```python
from build123d import *

# Parameters (mm, degrees)
BOSS_EXTRUDE3_DEPTH      = 6.35
FILLET1_R                = 6.35
CIRPATTERN5_COUNT        = 4
FILLET1_OF_CIRPATTERN5_R = 6.35
BOSS_EXTRUDE4_DEPTH      = 6.35
CIRPATTERN4_COUNT        = 4
SKETCH6_R                = 234.193665804
SKETCH6_R_2              = 215.9
CUT_EXTRUDE1_DEPTH       = 350.00288517
FILLET2_R                = 0.635
SKETCH7_R                = 60.93897947
CUT_EXTRUDE2_DEPTH       = 4.953
SKETCH8_R                = 79.670197019
CUT_EXTRUDE3_DEPTH       = 18.9484
CUT_EXTRUDE4_START       = 20.32
SKETCH11_R               = 219.71
SKETCH11_R_2             = 50.8
CUT_EXTRUDE4_DEPTH       = 20.32
CUT_EXTRUDE10_REACH      = 337.887
SKETCH20_R               = 30.226
SKETCH20_R_2             = 26.8224
CUT_EXTRUDE11_DEPTH      = 2.0066
CUT_EXTRUDE13_DEPTH      = 3.175
CIRPATTERN6_COUNT        = 8
SKETCH24_W               = 27.0002
SKETCH24_H               = 10.092146942
SKETCH25_R               = 27.9527
CUT_EXTRUDE14_DEPTH      = 14.3002


with BuildPart() as part:
    # Sketch1 → Revolve2 (revolve)
    with BuildSketch(Plane.XY, mode=Mode.PRIVATE) as revolve2_sk:
        with BuildLine():
            Line((-140.081298787, 50.8), (-140.081298787, 0))
            Line((-140.081298787, 0), (-39.979898787, 0))
            Line((-39.979898787, 0), (-39.979898787, 46.736))
            Line((-39.979898787, 46.736), (-43.154898787, 46.736))
            ThreePointArc((-43.154898787, 46.736), (-47.645026847, 48.595871939), (-49.504898787, 53.086))
            Line((-49.504898787, 53.086), (-49.504898787, 219.71))
            Line((-49.504898787, 219.71), (-64.998898787, 219.71))
            Line((-64.998898787, 219.71), (-64.998898787, 63.5))
            ThreePointArc((-64.998898787, 63.5), (-68.718642666, 54.519743879), (-77.698898787, 50.8))
            Line((-77.698898787, 50.8), (-140.081298787, 50.8))
        make_face()
        with BuildLine():
            Line((-9.677698787, 219.71), (-17.678698787, 219.71))
            Line((-17.678698787, 219.71), (-17.678698787, 77.7875))
            Line((-17.678698787, 77.7875), (1.650701213, 77.7875))
            Line((1.650701213, 77.7875), (18.846501213, 77.7875))
            Line((18.846501213, 77.7875), (18.846501213, 93.599))
            ThreePointArc((18.846501213, 93.599), (18.400131948, 94.676630735), (17.322501213, 95.123))
            Line((17.322501213, 95.123), (-6.629698787, 95.123))
            ThreePointArc((-6.629698787, 95.123), (-7.707329521, 95.569369265), (-8.153698787, 96.647))
            Line((-8.153698787, 96.647), (-8.153698787, 218.186))
            ThreePointArc((-8.153698787, 218.186), (-8.600068052, 219.263630735), (-9.677698787, 219.71))
        make_face()
    revolve(revolve2_sk.sketch.rotate(Axis((-140.081298787, 0, 0), (1, 0, 0)), 180), axis=Axis((-140.081298787, 0, 0), (1, 0, 0)))

    # Sketch4 → Boss-Extrude3 (add, symmetric)
    with BuildSketch(Plane(origin=(0, 0, 0), x_dir=(1, 0, 0), z_dir=(0, -0.7071067811865488, 0.7071067811865464))):
        Polygon((-17.678698787, 219.71), (-30.378698787, 219.71), (-30.378698787, 130.302), (-36.804898787, 130.302), (-36.804898787, 219.71), (-49.504898787, 219.71), (-49.504898787, 77.7875), (-17.678698787, 77.7875), align=None)
    boss_extrude3 = extrude(amount=BOSS_EXTRUDE3_DEPTH, both=True)

    # Fillet1
    # the kernel refuses this fillet: 6.35 mm, written as the material it takes off along each edge
    with BuildSketch(Plane(origin=(-30.378698787, 87.647299742, 96.627555863), x_dir=(0, -0.7071067811865464, -0.7071067811865486), z_dir=(-1, 0, 0))) as fillet1_piece_1:
        with BuildLine():
            CenterArc((FILLET1_R, -FILLET1_R), FILLET1_R, 90, 90)
            Line((0, -FILLET1_R), (0, 0))
            Line((0, 0), (FILLET1_R, 0))
        make_face()
    extrude(amount=6.4262, mode=Mode.SUBTRACT)
    with BuildSketch(Plane(origin=(-30.378698787, 96.627555863, 87.647299742), x_dir=(0, -0.7071067811865464, -0.7071067811865486), z_dir=(-1, 0, 0))) as fillet1_piece_2:
        with BuildLine():
            CenterArc((FILLET1_R, FILLET1_R), FILLET1_R, 180, 90)
            Line((0, FILLET1_R), (0, 0))
            Line((0, 0), (FILLET1_R, 0))
        make_face()
    extrude(amount=6.4262, mode=Mode.SUBTRACT)
    with BuildSketch(Plane(origin=(-49.504898787, 59.494196802, 50.513940681), x_dir=(0, 0.707106781186547, 0.7071067811865481), z_dir=(1, 0, 0)), Plane(origin=(-49.504898787, 50.513940681, 59.494196802), x_dir=(0, 0.7071067811865492, -0.7071067811865459), z_dir=(1, 0, 0))) as fillet1_piece_3:
        with BuildLine():
            CenterArc((FILLET1_R, FILLET1_R), FILLET1_R, 180, 90)
            Line((0, FILLET1_R), (0, 0))
            Line((0, 0), (FILLET1_R, 0))
        make_face()
    extrude(amount=31.8262, mode=Mode.SUBTRACT)

    # CirPattern5: Boss-Extrude3 ×4 about axis
    cirpattern5_axis = Axis((0, 0, 0), (1, 0, 0))
    for i in range(1, CIRPATTERN5_COUNT):
        add(boss_extrude3.rotate(cirpattern5_axis, i * 360 / CIRPATTERN5_COUNT))

    # Fillet1 of CirPattern5
    # the kernel refuses this fillet: 6.35 mm, written as the material it takes off along each edge
    with BuildSketch(Plane(origin=(-30.378698787, -96.627555863, 87.647299742), x_dir=(0, 0.7071067811865509, -0.7071067811865441), z_dir=(-1, 0, 0)), Plane(origin=(-30.378698787, -87.647299742, -96.627555863), x_dir=(0, 0.7071067811865452, 0.7071067811865498), z_dir=(-1, 0, 0)), Plane(origin=(-30.378698787, 96.627555863, -87.647299742), x_dir=(0, -0.7071067811865498, 0.7071067811865454), z_dir=(-1, 0, 0))) as fillet1_of_cirpattern5_piece_1:
        with BuildLine():
            CenterArc((FILLET1_OF_CIRPATTERN5_R, -FILLET1_OF_CIRPATTERN5_R), FILLET1_OF_CIRPATTERN5_R, 90, 90)
            Line((0, -FILLET1_OF_CIRPATTERN5_R), (0, 0))
            Line((0, 0), (FILLET1_OF_CIRPATTERN5_R, 0))
        make_face()
    extrude(amount=6.4262, mode=Mode.SUBTRACT)
    with BuildSketch(Plane(origin=(-30.378698787, -87.647299742, 96.627555863), x_dir=(0, 0.7071067811865509, -0.7071067811865441), z_dir=(-1, 0, 0)), Plane(origin=(-30.378698787, -96.627555863, -87.647299742), x_dir=(0, 0.7071067811865441, 0.7071067811865509), z_dir=(-1, 0, 0)), Plane(origin=(-30.378698787, 87.647299742, -96.627555863), x_dir=(0, -0.7071067811865509, 0.7071067811865441), z_dir=(-1, 0, 0))) as fillet1_of_cirpattern5_piece_2:
        with BuildLine():
            CenterArc((FILLET1_OF_CIRPATTERN5_R, FILLET1_OF_CIRPATTERN5_R), FILLET1_OF_CIRPATTERN5_R, 180, 90)
            Line((0, FILLET1_OF_CIRPATTERN5_R), (0, 0))
            Line((0, 0), (FILLET1_OF_CIRPATTERN5_R, 0))
        make_face()
    extrude(amount=6.4262, mode=Mode.SUBTRACT)
    with BuildSketch(Plane(origin=(-49.504898787, -50.513940681, 59.494196802), x_dir=(0, -0.7071067811865475, 0.7071067811865475), z_dir=(1, 0, 0)), Plane(origin=(-49.504898787, -59.494196802, 50.513940681), x_dir=(0, 0.7071067811865464, 0.7071067811865486), z_dir=(1, 0, 0)), Plane(origin=(-49.504898787, -59.494196802, -50.513940681), x_dir=(0, -0.7071067811865481, -0.707106781186547), z_dir=(1, 0, 0)), Plane(origin=(-49.504898787, -50.513940681, -59.494196802), x_dir=(0, -0.7071067811865486, 0.7071067811865464), z_dir=(1, 0, 0)), Plane(origin=(-49.504898787, 50.513940681, -59.494196802), x_dir=(0, 0.7071067811865476, -0.7071067811865476), z_dir=(1, 0, 0)), Plane(origin=(-49.504898787, 59.494196802, -50.513940681), x_dir=(0, -0.7071067811865459, -0.7071067811865492), z_dir=(1, 0, 0))) as fillet1_of_cirpattern5_piece_3:
        with BuildLine():
            CenterArc((FILLET1_OF_CIRPATTERN5_R, FILLET1_OF_CIRPATTERN5_R), FILLET1_OF_CIRPATTERN5_R, 180, 90)
            Line((0, FILLET1_OF_CIRPATTERN5_R), (0, 0))
            Line((0, 0), (FILLET1_OF_CIRPATTERN5_R, 0))
        make_face()
    extrude(amount=31.8262, mode=Mode.SUBTRACT)

    # Sketch5 → Boss-Extrude4 (add, symmetric)
    with BuildSketch(Plane(origin=(0, 0, 0), x_dir=(-1, 0, 0), z_dir=(0, 0, -1))):
        Polygon((49.504898787, 219.71), (49.504898787, 73.66), (36.804898787, 86.36), (36.804898787, 219.71), align=None)
        Polygon((17.678698787, 77.7875), (17.678698787, 219.71), (30.378698787, 219.71), (30.378698787, 90.4875), align=None)
    boss_extrude4 = extrude(amount=BOSS_EXTRUDE4_DEPTH, both=True)

    # CirPattern4: Boss-Extrude4 ×4 about axis
    cirpattern4_axis = Axis((0, 0, 0), (1, 0, 0))
    for i in range(1, CIRPATTERN4_COUNT):
        add(boss_extrude4.rotate(cirpattern4_axis, i * 360 / CIRPATTERN4_COUNT))

    # Sketch6 → Cut-Extrude1 (cut, through all)
    with BuildSketch(Plane.ZY.offset(140.081298787)):
        Circle(SKETCH6_R)
        with Locations(Location((0, 0, 0), (0, 0, 270))):
            Circle(SKETCH6_R_2, mode=Mode.SUBTRACT)
    extrude(amount=-CUT_EXTRUDE1_DEPTH, mode=Mode.SUBTRACT)

    # Fillet2
    fillet2_edges = [part.edges().sort_by_distance(p)[0] for p in [
        (-39.979898787, 46.736, 0),
    ]]
    fillet(fillet2_edges, radius=FILLET2_R)

    # Sketch7 → Cut-Extrude2 (cut)
    with BuildSketch(Plane(origin=(-39.979898787, 0, 0), x_dir=(0, 0, -1), z_dir=(1, 0, 0))):
        Circle(SKETCH7_R)
    extrude(amount=-CUT_EXTRUDE2_DEPTH, mode=Mode.SUBTRACT)

    # Sketch8 → Cut-Extrude3 (cut)
    with BuildSketch(Plane.ZY.offset(140.081298787)):
        Circle(SKETCH8_R)
    extrude(amount=-CUT_EXTRUDE3_DEPTH, mode=Mode.SUBTRACT)

    # Sketch11 → Cut-Extrude4 (cut)
    with BuildSketch(Plane.ZY.offset(64.998898787).offset(CUT_EXTRUDE4_START)):
        Circle(SKETCH11_R)
        with Locations(Location((0, 0, 0), (0, 0, 270))):
            Circle(SKETCH11_R_2, mode=Mode.SUBTRACT)
    extrude(amount=-CUT_EXTRUDE4_DEPTH, mode=Mode.SUBTRACT)

    # Sketch12 → Cut-Revolve1 (revolve, cut)
    with BuildSketch(Plane(origin=(0, 0, 0), x_dir=(1, 0, 0), z_dir=(0, 1, 0)), mode=Mode.PRIVATE) as cut_revolve1_sk:
        with BuildLine():
            Line((-121.132898787, 31.75), (-80.111898787, 31.75))
            ThreePointArc((-80.111898787, 31.75), (-76.957987839, 32.588616713), (-74.637123327, 34.882961973))
            Line((-74.637123327, 34.882961973), (-65.874123327, 49.795890249))
            ThreePointArc((-65.874123327, 49.795890249), (-65.613530636, 50.287482958), (-65.396970658, 50.8))
            Line((-65.396970658, 50.8), (-121.132898787, 50.8))
            Line((-121.132898787, 50.8), (-121.132898787, 31.75))
        make_face()
    revolve(cut_revolve1_sk.sketch.rotate(Axis((-60.172898787, 0, 0), (-1, 0, 0)), 270), axis=Axis((-60.172898787, 0, 0), (-1, 0, 0)), mode=Mode.SUBTRACT)

    # Sketch18 → Cut-Extrude10 (cut, up to next)
    with BuildSketch(Plane.ZY.offset(121.132898787), mode=Mode.PRIVATE) as cut_extrude10_sk1:
        with BuildLine():
            Line((-14.359429538, -21.094621628), (-21.094621628, -14.359429538))
            Line((-21.094621628, -14.359429538), (-17.575856913, -10.840664823))
            ThreePointArc((-17.575856913, -10.840664823), (14.601896453, 14.601896453), (-10.840664823, -17.575856913))
            Line((-10.840664823, -17.575856913), (-14.359429538, -21.094621628))
        make_face()
    cut_extrude10_tool1 = extrude(cut_extrude10_sk1.sketch, amount=-CUT_EXTRUDE10_REACH, mode=Mode.PRIVATE) & part.part
    add(cut_extrude10_tool1.solids().sort_by_distance((-121.132899, -0.51024, -0.51024))[0], mode=Mode.SUBTRACT)

    # Sketch20 → Cut-Extrude11 (cut)
    with BuildSketch(Plane.ZY.offset(121.132898787)):
        with Locations(Location((0, 0, 0), (0, 0, 270))):
            Circle(SKETCH20_R)
        with Locations(Location((0, 0, 0), (0, 0, 270))):
            Circle(SKETCH20_R_2, mode=Mode.SUBTRACT)
    extrude(amount=-CUT_EXTRUDE11_DEPTH, mode=Mode.SUBTRACT)

    # Sketch22 → Cut-Extrude13 (cut)
    with BuildSketch(Plane.ZY.offset(64.998898787)):
        with BuildLine():
            Line((50.92871008, 64.399094261), (145.78051919, 159.250903372))
            ThreePointArc((145.78051919, 159.250903372), (82.621353048, 199.465591069), (9.525, 215.689787368))
            Line((9.525, 215.689787368), (9.525, 84.123223233))
            ThreePointArc((9.525, 84.123223233), (24.00104092, 61.192302667), (50.92871008, 64.399094261))
        make_face()
    cut_extrude13 = extrude(amount=-CUT_EXTRUDE13_DEPTH, mode=Mode.SUBTRACT)

    # CirPattern6: Cut-Extrude13 ×8 about axis
    cirpattern6_axis = Axis((0, 0, 0), (1, 0, 0))
    for i in range(1, CIRPATTERN6_COUNT):
        add(cut_extrude13.rotate(cirpattern6_axis, i * 360 / CIRPATTERN6_COUNT), mode=Mode.SUBTRACT)

    # Sketch24 → Cut-Revolve2 (revolve, cut)
    with BuildSketch(Plane(origin=(0, 0, 0), x_dir=(1, 0, 0), z_dir=(0, 1, 0)), mode=Mode.PRIVATE) as cut_revolve2_sk:
        with Locations((5.346401213, 95.533573471)):
            Rectangle(SKETCH24_W, SKETCH24_H)
    revolve(cut_revolve2_sk.sketch.rotate(Axis((-154.951085714, 0, 0), (1, 0, 0)), 271.68541304), axis=Axis((-154.951085714, 0, 0), (1, 0, 0)), mode=Mode.SUBTRACT)

    # Sketch25 → Cut-Extrude14 (cut)
    with BuildSketch(Plane(origin=(-44.932898787, 0, 0), x_dir=(0, 0, -1), z_dir=(1, 0, 0))):
        with Locations(Location((0, 0, 0), (0, 0, 90))):
            Circle(SKETCH25_R)
    extrude(amount=-CUT_EXTRUDE14_DEPTH, mode=Mode.SUBTRACT)


solid = part.part
```
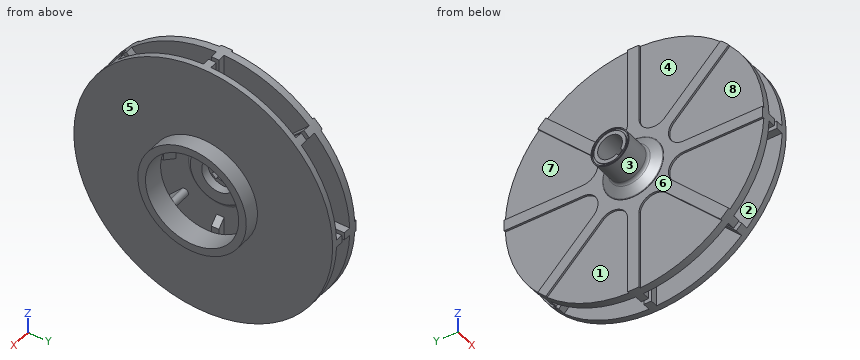
Could you check a few things on this model? Use its own coordinates, in mm. Face numbers are marked on the shaded views. A direction names the side the tool comes from. Round coordinates to 2 decimals unless told otherwise and drop trailing zeros. Write each loop counter-clockwise with the first axis right and the second up, starting at its lowest first coordinate (ties: lowest second). Pieces come first, ordered by that corner, then holes. Notation, with made-up numbers: M -3.75,58.25 L 3.25,58.25 A33 ccw 3.25,86.25 Z; hole C -9,-29.5 d10. An arc over 180 degrees is marked long. Write each question's results on one line, items separated by ' | '. Start each with the question number.
1. I'm going to push flat-ended pins straight in: pin 1 Ø10 at (x, z) = (-46, -135.5) entering from +Y; pin 2 Ø12 at (y, z) = (160.5, -88.5) entering from +X; pin 3 Ø5 at (y, z) = (-131.5, 32.5) entering from -X. Where does each tip first touch, or does it pass through?
2. Imagine slicing it at B-B on x = 3. List the corners of the cut face in (y, z) for me (1 decimal), and give its area (3 significant figures).
3. On a 3-axis mill with a long thin cutter (end or side, diameter ignored), from which of +Z, -Z, +X, -X, +Y, -Y can I reach the whole of each face in a straight line? I mean the marked faces 4, 5, 6, 7 and 8. Say none if no direction works.
4. Thinking about a two-plate mould opening in X: for the marked faces 1, 2 and 3, which applies, +X half, -X half, draft (parallel to the pull), parting line (faces both ways), or undercut?
5. I need wall thicknesses on L1, parallel to X at y = -175, z = 65; L2, parallel to X at y = 148, z = 156; L3, parallel to Z at x = -4.5, y = 0. Which ranges of each line are inside material? Lowest first, please. Write a range as from..to.
6. Imagine slicing it at A-A on z = -188. List the corners of the cut face in (x, y) for me (3 decimals), and give its area (3 significant figures).
Result sheet:
1) pin 1: stops at y = 170.9 | pin 2: stops at x = -8.15 | pin 3: stops at x = -61.82
2) outline: C 0,0 d181; hole C 0,0 d155.6 | area: 6,710 mm^2
3) face 4: +Z, -X | face 5: +X | face 6: -X | face 7: -X, +Y | face 8: -X, -Y
4) face 1: -X half | face 2: undercut | face 3: draft
5) L1: x = -61.82..-49.5, -17.68..-8.15 | L2: x = -65..-36.8, -30.38..-8.15 | L3: z = -90.49..-77.79, 77.79..90.49
6) outline: M -64.999,-9.525 L -61.824,-9.525 L -61.824,-106.155 L -49.505,-106.155 L -49.505,-6.35 L -36.805,-6.35 L -36.805,6.35 L -49.505,6.35 L -49.505,106.155 L -61.824,106.155 L -61.824,9.525 L -64.999,9.525 Z; M -30.379,-6.35 L -17.679,-6.35 L -17.679,-106.155 L -8.154,-106.155 L -8.154,106.155 L -17.679,106.155 L -17.679,6.35 L -30.379,6.35 Z | area: 5,020 mm^2
